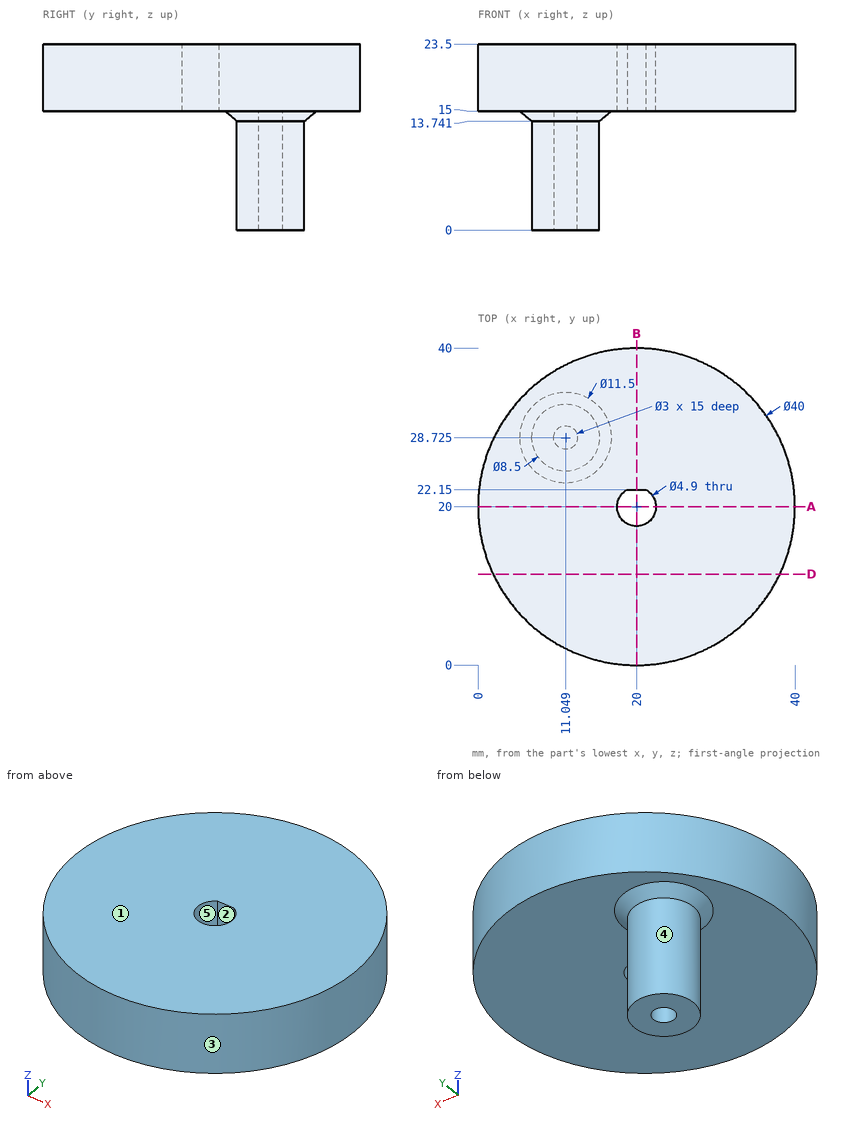
Study the drawing (mm; zero at the part's minimum x, y, z) and answer. A direction names the side the tool comes from. Coordinates: 2 decimals unless noted, no trailing zeros. Write each loop counter-clockwise with the first axis right and the second up, starting at its lowest first coordinate (ties: lowest second). Pieces come first, ordered by that corner, then holes. Notation, with made-up numbers: (-8, 6) - (35, 6) arc R21 ccw to (35, 28) - close; hole circle Ø7 at (67.5, 74). An arc over 180 degrees is marked (long way). Answer as a JSON object with one key per item and string values. Group by question number.
1. Which of the six approach directions +Z, -Z, +X, -X, +Y, -Y give full straight-line access (tool end or side, diameter ignored) to the marked faces 4 and 5?
2. The mould has two halves that part along Y. Classify the marked faces 1, 2 and 3: +Y half, -Y half, draft (parallel to the pull), parting line (faces both ways), or undercut.
3. Each of these flat-tipped pins is pushed along its axis until it touches: P1, Ø1.2, axis at x = 19.5, z = 18, coming from the -Y side; P2, Ø10, axis at x = 13, z = 14.5, coming from the -Y side; P3, Ø5, axis at x = 20.5, y = 18, coming from the -Z side. Where does it stop, or does it pass through?
4. Consider L1, parallel to Z at x = 20.5, y = 34; L2, parallel to Y at x = 20, z = 20.25; L3, parallel to Y at x = 12, z = 8.5 (1 decimal). Determine where each line is inside the solid, lowest interval first. Write a range as [from, to].
5. A cutting plane is placed at D-D (y = 11.5). Determine the outline of the cut face in (x, z), plus the area to 3 significant figures.
6. A cutting plane is placed at B-B (x = 20). Determine the outline of the cut face in (y, z).
7. A cutting plane is placed at A-A (y = 20). Determine the outline of the cut face in (x, z).
Worked out:
{
 "1": {"face 4": "-Z", "face 5": "+Z, -Z"},
 "2": {"face 1": "draft", "face 2": "undercut", "face 3": "parting line"},
 "3": {"P1": "stops at y = 0", "P2": "stops at y = 0.1", "P3": "stops at z = 15"},
 "4": {"L1": "z = [15, 23.5]", "L2": "y = [0, 17.55], [22.15, 40]", "L3": "y = [24.6, 27.6], [29.9, 32.9]"},
 "5": {"outline": "(1.9, 15) - (38.1, 15) - (38.1, 23.5) - (1.9, 23.5) - close", "area": "308 mm²"},
 "6": {"outline": "(0, 15) - (17.55, 15) - (17.55, 23.5) - (0, 23.5) - close; (22.15, 15) - (40, 15) - (40, 23.5) - (22.15, 23.5) - close"},
 "7": {"outline": "(0, 15) - (17.55, 15) - (17.55, 23.5) - (0, 23.5) - close; (22.45, 15) - (40, 15) - (40, 23.5) - (22.45, 23.5) - close"}
}
